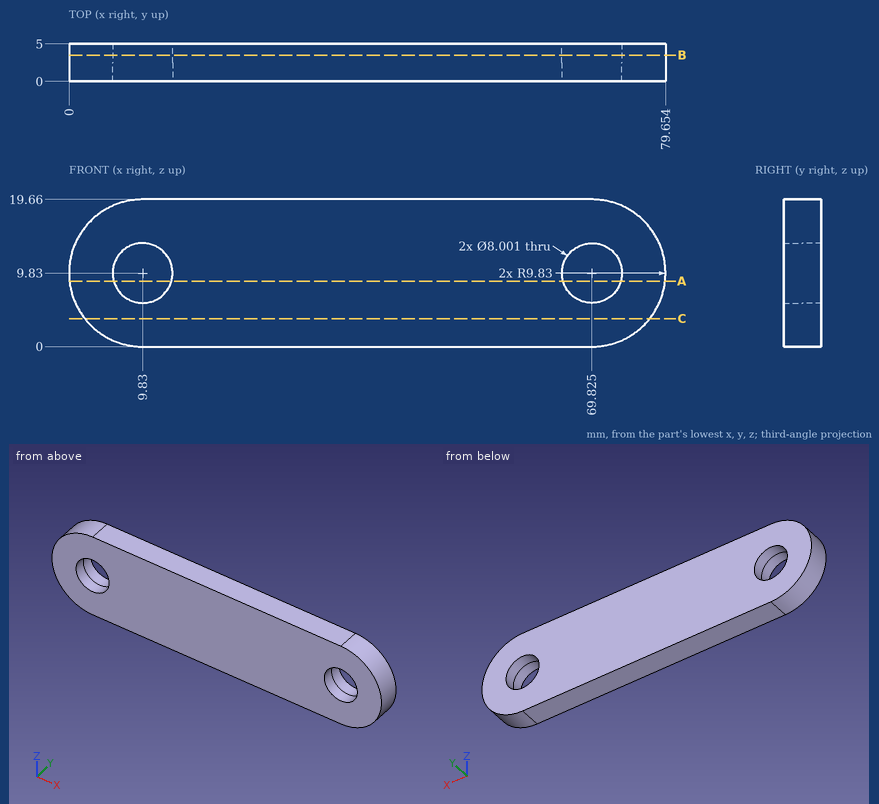
Drawing for the job (mm, zero at the part's lowest x, y, z). Round coordinates to 2 decimals unless told otherwise and drop trailing zeros. Loops run counter-clockwise (first coordinate to the right, second up) from the corner with the lowest first, then second, coordinate; pieces in that order, holes last. Notation, with made-up numbers: M 85.5,40 L 91.5,40 A17 cw 91.5,57 Z; hole C -18,0.25 d8. An arc over 180 degrees is marked long. Use a Markdown table: item, result. Add a question column.
(1) Drill centre lines: line 1 (X direction, y = 3.9, z = 9.75) (1 decimal); line 2 (X direction, y = 3.3, z = 11.75) (1 decimal); line 3 (Z direction, x = 67.5, y = 1.5) (1 decimal). Where is each one in solid material? Low to high.
(2) Cut at C-C (z = 3.75). Give the cut face in (x, y) (1 decimal).
(3) Cut at B-B (y = 3.5). Give the cut face in (x, z) (1 decimal).
(4) Cut at A-A (z = 8.75). Give the cut face in (x, y) (1 decimal), and give its area (3 significant figures).
Geometry says:
| question | item | result |
|---|---|---|
| 1 | line 1 | x = 0 to 5.8, 13.8 to 65.8, 73.8 to 79.7 |
| 1 | line 2 | x = 0.2 to 6.3, 13.3 to 66.3, 73.3 to 79.5 |
| 1 | line 3 | z = 0 to 6.6, 13.1 to 19.7 |
| 2 | outline | M 2.1,0 L 77.5,0 L 77.5,5 L 2.1,5 Z |
| 3 | outline | M 9.8,0 L 69.8,0 A9.8 ccw 69.8,19.7 L 9.8,19.7 A9.8 ccw Z; hole C 9.8,9.8 d8; hole C 69.8,9.8 d8 |
| 4 | outline | M 0.1,0 L 6,0 L 6,5 L 0.1,5 Z; M 13.7,0 L 66,0 L 66,5 L 13.7,5 Z; M 73.7,0 L 79.6,0 L 79.6,5 L 73.7,5 Z |
| 4 | area | 321 mm² |
